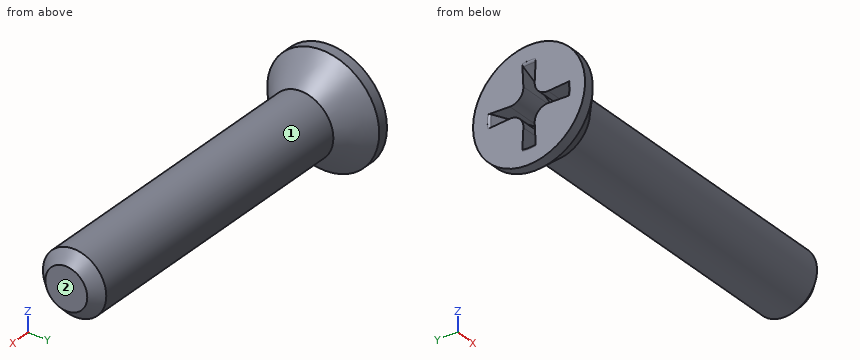
Autodesk Inventor part; units mm, degrees
ref_plane "Work Plane2" through (2.032, 0, 0) normal (0, 1, 0) x (1, 0, 0)
ref_plane "YZ Plane" through (0, 0, 0) normal (1, 0, 0) x (0, 1, 0)
ref_plane "XZ Plane" through (0, 0, 0) normal (0, 1, 0) x (-1, 0, 0)
sketch "Sketch1" plane through (0, 0, 0) normal (0, 0, 1) x (1, 0, 0)
  line L0 (2.6924, 0) -> (19.05, 0)
  line L1 (19.05, 0) -> (19.05, 1.7526)
  line L2 (19.05, 1.7526) -> (2.1082, 1.7526)
  line L3 (0.5596, 3.0988) -> (0, 3.0988)
  line L4 (-3.81, 0) -> (22.86, 0)
  line L5 (0, -0.6198) -> (0, 3.7186)
  line L6 (0, 2.2098) -> (2.0648, 1.1803)
  line L7 (2.0648, 1.1803) -> (2.6924, 0)
  line L8 (2.1082, 1.7526) -> (0.5596, 3.0988)
  line L9 (0, 3.0988) -> (0, 2.2098)
  dimension "d2" = 3.5052
  dimension "d3" = 6.1976
  dimension "d4" = 2.6924
  dimension "d5" = 4.4196
  dimension "d6" = 26.5
  dimension "d7" = 62
  dimension "d13" = 41
  dimension "d14" = 2.1082
  dimension "d15" = 19.05
revolve "Body" add sketch "Sketch1" angle 360 about axis through (2.6924, 0, 0) along (1, 0, 0) contours L7 L6 L5 L3 L8 L2 L1 L0
sketch "Sketch2" plane through (0, 0, 0) normal (-1, 0, 0) x (0, 0, 1)
  line L0 (0, -4.3383) -> (0, 4.3383)
  line L1 (-4.3383, 0) -> (4.3383, 0)
  line L2 (0, 2.2098) -> (0, 0) construction
  line L3 (0, 0) -> (2.2098, 0) construction
  arc A0 (0.7366, 0) -> (0, 0.7366) centre (0, 0) ccw
  line L4 (0, 0) -> (0.7947, 0.7947) construction
  arc A1 (1.1049, 0) -> (0, 1.1049) centre (0, 0) ccw construction
  line L5 (0.3683, 2.1789) -> (0.3131, 1.0596)
  line L6 (2.1789, 0.3683) -> (1.0596, 0.3131)
  arc A2 (0.3131, 1.0596) -> (1.0596, 0.3131) centre (1.0245, 1.0245) ccw
  arc A3 (2.2098, 0) -> (2.1789, 0.3683) centre (0, 0) ccw
  arc A4 (0.3683, 2.1789) -> (0, 2.2098) centre (0, 0) ccw
  arc A5 (2.1789, 0.3683) -> (0.3683, 2.1789) centre (0, 0) ccw
  line L7 (0.3683, -2.1789) -> (0.3131, -1.0596)
  line L8 (2.1789, -0.3683) -> (1.0596, -0.3131)
  arc A6 (1.0596, -0.3131) -> (0.3131, -1.0596) centre (1.0245, -1.0245) ccw
  arc A7 (2.1789, -0.3683) -> (2.2098, 0) centre (0, 0) ccw
  arc A8 (0, -2.2098) -> (0.3683, -2.1789) centre (0, 0) ccw
  arc A9 (0.3683, -2.1789) -> (2.1789, -0.3683) centre (0, 0) ccw
  line L9 (-0.3683, 2.1789) -> (-0.3131, 1.0596)
  line L10 (-2.1789, 0.3683) -> (-1.0596, 0.3131)
  arc A10 (-1.0596, 0.3131) -> (-0.3131, 1.0596) centre (-1.0245, 1.0245) ccw
  arc A11 (-2.1789, 0.3683) -> (-2.2098, 0) centre (0, 0) ccw
  arc A12 (0, 2.2098) -> (-0.3683, 2.1789) centre (0, 0) ccw
  arc A13 (-0.3683, 2.1789) -> (-2.1789, 0.3683) centre (0, 0) ccw
  arc A14 (-2.1789, -0.3683) -> (-0.3683, -2.1789) centre (0, 0) ccw
  arc A15 (-0.3683, -2.1789) -> (0, -2.2098) centre (0, 0) ccw
  arc A16 (-2.2098, 0) -> (-2.1789, -0.3683) centre (0, 0) ccw
  line L11 (-2.1789, -0.3683) -> (-1.0596, -0.3131)
  arc A17 (-0.3131, -1.0596) -> (-1.0596, -0.3131) centre (-1.0245, -1.0245) ccw
  line L12 (-0.3683, -2.1789) -> (-0.3131, -1.0596)
  dimension "d18" = 45
  dimension "d19" = 1.4732
  dimension "d20" = 2.2098
  dimension "d21" = 4.4196
  dimension "d22" = 0.3683
extrude "Slot" add sketch "Sketch2" against normal up to next contours A2 L5 A5 L6 | L9 A10 L10 A13 | L7 A6 L8 A9 | A14 L11 A17 L12
fillet "Fillet1" radius 0.1473 4 edges at (0, 2.2098, 0) (0, 0, 2.2098) (0, -2.2098, 0) (0, 0, -2.2098)
thread "Thread"
chamfer "Chamfer1" distance 0.5953 distance2 0.5953 1 edges at (19.05, -1.7526, 0) measured on face at (19.05, -0.3126, 0.4528)
ref_plane "Work Plane2" through (2.032, 0, 0) normal (0, 1, 0) x (1, 0, 0)
equation "\"d2\" = GD"
equation "\"d3\" = KOD"
equation "\"d4\" = INTI"
equation "\"d5\" = SDM"
equation "\"d13\" = 0.5 * SEWI"
equation "\"d14\" = KOH"
equation "\"d15\" = NLG"
equation "\"d19\" = 0.333333 * SDM"
equation "\"d20\" = 0.5 * SDM"
equation "\"d21\" = SDM"
equation "\"d22\" = 0.5 * SBR"
equation "\"d45\" = INTI"
equation "\"d25\" = 0.2 * SBR"
equation "\"d9\" = GEL"
equation "\"d11\" = -0.5 * SPD + 0.5 * GD"
equation "\"d12\" = GUL"
equation "\"GD\" = NND"
equation "\"NLG\" = 19.05"
equation "\"GEL\" = 14.95743"
equation "\"KOD\" = 6.1976"
equation "\"KOH\" = 2.1082"
equation "\"SDM\" = 4.4196"
equation "\"INTI\" = 2.6924"
equation "\"SBR\" = 0.7366"
equation "\"GUL\" = 0.75 * GAL"
equation "\"SPD\" = 2.31458"
equation "\"SEWI\" = 82deg"
equation "\"d0\" = NLG"
equation "\"d1\" = KOH"
equation "\"d17\" = SDM"
equation "\"TOA\" = 30deg"
equation "\"THREADDIA\" = 3.5052"
equation "\"BDM\" = NND"
equation "\"NND\" = 3.5052"
equation "\"GAL\" = 0.79375"
equation "\"GD1\" = SPD"
properties part number "ANSI B18.6.3 - 6-32 x 3/4, CRFCHMSTII(5)" material "Steel, Mild"
Here's how the part is built. I have some questions about the finished solid (model axes, mm). Face numbers are marked on the shaded views. A direction names the side the tool comes from. Coordinates: 2 decimals unless noted, no trailing zeros. Write each loop counter-clockwise with the first axis right and the second up, starting at its lowest first coordinate (ties: lowest second). Pieces come first, ordered by that corner, then holes. Notation, with made-up numbers: (8, -15) -> (13, -15) arc R28 ccw to (13, 14) -> close; hole circle Ø9 at (-25, 82). An arc over 180 degrees is marked (long way). Use a Markdown table: item, result. Add a question column.
(1) I'm going to push flat-ended pins straight in: P1, Ø1.5, axis at x = 7.5, z = -2, coming from the -Y side; P2, Ø3, axis at x = 13, z = 0, coming from the +Y side; P3, Ø1.5, axis at x = 8, z = -1, coming from the -Y side. Where does each tip first touch, or does it pass through?
(2) For the marked faces 1 and 2, which set-ups out of +Z, -Z, +X, -X, +Y, -Y let a thin tool reach every point of the face, with its end or its side?
(3) Please list where these lines run through material, in increasing order: line 1 (X direction, y = 1, z = -1); line 2 (Z direction, x = 10.75, y = 0.5); line 3 (X direction, y = 1.75, z = -1.5).
(4) If we section it at A-A, the plane x = 2.5: Write out the boundary of the cut face in (y, z).
Outcome:
| question | item | result |
|---|---|---|
| 1 | P1 | stops at y = -1.23 |
| 1 | P2 | stops at y = 1.75 |
| 1 | P3 | stops at y = -1.73 |
| 2 | face 1 | +X |
| 2 | face 2 | +Z, -Z, +X, +Y, -Y |
| 3 | line 1 | x = 0 to 18.79 |
| 3 | line 2 | z = -1.68 to 1.68 |
| 3 | line 3 | x = 0 to 1.47 |
| 4 | outline | circle Ø3.51 at (0, 0); hole circle Ø0.72 at (0, 0) |
